```python
from build123d import *

# Parameters (mm, degrees)
BOSS_EXTRUDE1_DEPTH = 5.842
FILLET1_R           = 1.5875
SKETCH2_R           = 2.38125
CUT_EXTRUDE1_DEPTH  = 38.14766282


with BuildPart() as part:
    # Sketch1 → Boss-Extrude1 (new body)
    with BuildSketch(Plane(origin=(0, 0, 0), x_dir=(1, 0, 0), z_dir=(0, 1, 0))):
        Polygon((-25.4, -12.7), (25.4, -12.7), (25.4, -6.35), (31.242, -6.35), (31.242, -9.525), (34.417, -9.525), (34.417, 9.525), (31.242, 9.525), (31.242, 6.35), (25.4, 6.35), (25.4, 12.7), (-25.4, 12.7), (-25.4, 6.35), (-31.242, 6.35), (-31.242, 9.525), (-34.417, 9.525), (-34.417, -9.525), (-31.242, -9.525), (-31.242, -6.35), (-25.4, -6.35), align=None)
    extrude(amount=BOSS_EXTRUDE1_DEPTH)

    # Fillet1
    fillet1_edges = [part.edges().sort_by_distance(p)[0] for p in [
        (34.417, 2.921, -9.525),
        (34.417, 2.921, 9.525),
        (-34.417, 2.921, 9.525),
        (-34.417, 2.921, -9.525),
    ]]
    fillet(fillet1_edges, radius=FILLET1_R)

    # Sketch2 → Cut-Extrude1 (cut, through all)
    with BuildSketch(Plane(origin=(0, 5.842, 0), x_dir=(1, 0, 0), z_dir=(0, 1, 0))):
        with Locations(Location((0, 0, 0), (0, 0, 270))):
            Circle(SKETCH2_R)
        with Locations(Location((12.7, 0, 0), (0, 0, 270))):
            Circle(SKETCH2_R)
        with Locations(Location((-12.7, 0, 0), (0, 0, 90))):
            Circle(SKETCH2_R)
    extrude(amount=-CUT_EXTRUDE1_DEPTH, mode=Mode.SUBTRACT)


solid = part.part
```
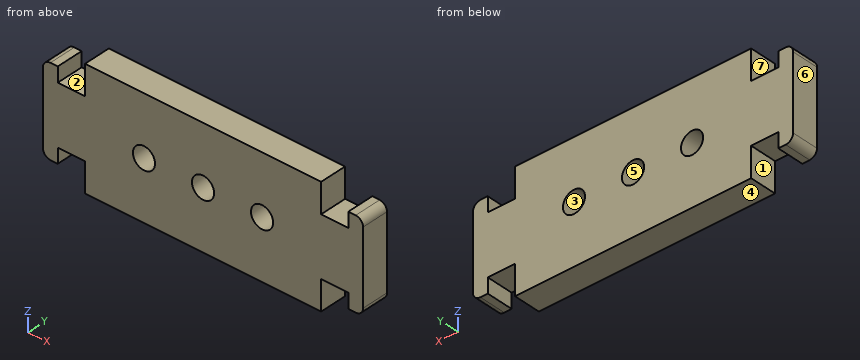
The model under review builds one solid part; all positions refer to its coordinate system, in mm. Face numbers are marked on the shaded views. A direction names the side the tool comes from. Round coordinates to 2 decimals unless told otherwise and drop trailing zeros. Loops run counter-clockwise (first coordinate to the right, second up) from the corner with the lowest first, then second, coordinate; pieces in that order, holes last. Notation, with made-up numbers: M 88.5,-23.75 L 95.5,-23.75 A27 ccw 95.5,0.25 Z; hole C 63.5,-2.75 d9. An arc over 180 degrees is marked long. Answer as a JSON object with one key per item and string values.
(1) Take a section at C-C on x = -12.7. Give the boundary of the cut face in (y, z), and give its area (3 significant figures).
Resolved:
{"outline": "M 0,-12.7 L 5.84,-12.7 L 5.84,-2.38 L 0,-2.38 Z; M 0,2.38 L 5.84,2.38 L 5.84,12.7 L 0,12.7 Z", "area": "121 mm²"}
(2) Clearance check with flat-ended pins moving along their axes: P1, Ø0.5, axis at x = -32.5, y = 4, coming from the -Z side (3 decimals); P2, Ø0.5, axis at x = 32, y = 1.5, coming from the +Z side (3 decimals); P3, Ø3, axis at x = 29, y = 2, coming from the -Z side. State where each tip first meets the part, or that it passes through.
Resolved:
{"P1": "z = -9.525", "P2": "z = 9.525", "P3": "z = -6.35"}
(3) To check wall thickness, follow line 1 along X through (y, z) = (2.65, 0); line 2 along X through (y, z) = (0.85, 6.5); line 3 along Z through (x, y) = (-12.7, 3.2). State the ranges of each line that lie inside material, in increasing order.
Resolved:
{"line 1": "-34.42 to -15.08, -10.32 to -2.38, 2.38 to 10.32, 15.08 to 34.42", "line 2": "-34.42 to -31.24, -25.4 to 25.4, 31.24 to 34.42", "line 3": "-12.7 to -2.38, 2.38 to 12.7"}
(4) Take a section at A-A on z = 0. Give the boundary of the cut face in (x, y), and give its area (3 significant figures).
Resolved:
{"outline": "M -34.42,0 L -15.08,0 L -15.08,5.84 L -34.42,5.84 Z; M -10.32,0 L -2.38,0 L -2.38,5.84 L -10.32,5.84 Z; M 2.38,0 L 10.32,0 L 10.32,5.84 L 2.38,5.84 Z; M 15.08,0 L 34.42,0 L 34.42,5.84 L 15.08,5.84 Z", "area": "319 mm²"}
(5) Tool access review of the marked faces 1, 2 and 3: name each direction out of +Z, -Z, +X, -X, +Y, -Y from which nothing blocks a thin tool from reaching the whole face with its end or side.
Resolved:
{"face 1": "-Z, +Y, -Y", "face 2": "+Z, +Y, -Y", "face 3": "+Y, -Y"}
(6) Take a section at B-B on y = 4.7. Count the separate pieces of the cut face and the enclosed holes in it, and give its area (3 significant figures).
Resolved:
{"separate pieces": "1", "enclosed holes": "3", "area": "1,500 mm²"}
(7) Take a section at D-D on z = 8.75. Give the boundary of the cut face in (x, y), and give its area (3 significant figures).
Resolved:
{"outline": "M -34.19,0 L -31.24,0 L -31.24,5.84 L -34.19,5.84 Z; M -25.4,0 L 25.4,0 L 25.4,5.84 L -25.4,5.84 Z; M 31.24,0 L 34.19,0 L 34.19,5.84 L 31.24,5.84 Z", "area": "331 mm²"}
(8) Draft analysis for pull direction X (two halves, no side actions). For the marked faces 4, 5, 6 and 7, state which applies: released by +X, released by -X, zero draft, split by the parting line, or undercut.
Resolved:
{"face 4": "zero draft", "face 5": "undercut", "face 6": "released by -X", "face 7": "undercut"}
